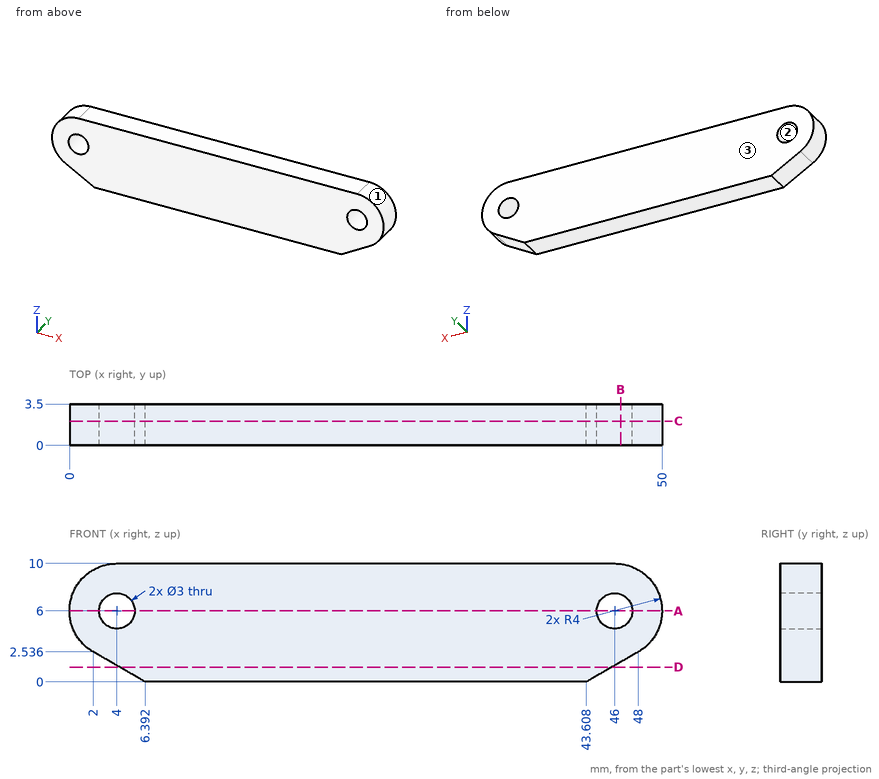
Source: three-view drawing plus pictorial views. Frame: mm from the lowest corner of the part. Coordinates: 2 decimals unless noted, no trailing zeros. Order: outer loops, then holes, each group sorted by start corner. A loop starts at its lowest first (then second) coordinate and runs counter-clockwise, first axis right, second up. Notation, with made-up numbers: M 31,-25.5 L 71,-25.5 A22 cw 71,7.5 Z; hole C 31,37 d9. An arc over 180 degrees is marked long. Answer in a Markdown table with one row per item.
(1) Contact query for a flat-ended pin moving along its axis: pin 1 Ø2 at (y, z) = (0.5, 7.5) entering from -X. Output: stop coordinate, or through.
Numbers:
| item | result |
|---|---|
| pin 1 | stops at x = 0.03 |
(2) Section query A-A, the plane z = 6. Output: boundary loops of the cut face in (x, y), plus the area to 3 significant figures.
Numbers:
| item | result |
|---|---|
| outline | M 0,0 L 2.5,0 L 2.5,3.5 L 0,3.5 Z; M 5.5,0 L 44.5,0 L 44.5,3.5 L 5.5,3.5 Z; M 47.5,0 L 50,0 L 50,3.5 L 47.5,3.5 Z |
| area | 154 mm^2 |
(3) Section query C-C, the plane y = 2.05. Output: boundary loops of the cut face in (x, z).
Numbers:
| item | result |
|---|---|
| outline | M 2,2.54 L 6.39,0 L 43.61,0 L 48,2.54 A4 ccw 46,10 L 4,10 A4 ccw Z; hole C 4,6 d3; hole C 46,6 d3 |
(4) Section query B-B, the plane x = 46.5. Output: boundary loops of the cut face in (y, z).
Numbers:
| item | result |
|---|---|
| outline | M 0,1.67 L 3.5,1.67 L 3.5,4.59 L 0,4.59 Z; M 0,7.41 L 3.5,7.41 L 3.5,9.97 L 0,9.97 Z |
(5) Material intervals for line 1 (X direction, y = 1.15, z = 6); line 2 (Z direction, x = 4, y = 1.9); line 3 (Z direction, x = 45, y = 2.15) (1 decimal), sorted ascending. Write a range as [from, to].
Numbers:
| item | result |
|---|---|
| line 1 | x = [0, 2.5], [5.5, 44.5], [47.5, 50] |
| line 2 | z = [1.38, 4.5], [7.5, 10] |
| line 3 | z = [0.8, 4.9], [7.1, 10] |
(6) Draft query along Z for the marked faces 1, 2 and 3. Return one class per face: pulls with the +Z half, pulls with the -Z half, needs draft (parallel to the pull), parting line crosses it, or undercut.
Numbers:
| item | result |
|---|---|
| face 1 | parting line crosses it |
| face 2 | undercut |
| face 3 | needs draft |
(7) Section query D-D, the plane z = 1.25. Output: boundary loops of the cut face in (x, y).
Numbers:
| item | result |
|---|---|
| outline | M 4.23,0 L 45.77,0 L 45.77,3.5 L 4.23,3.5 Z |
